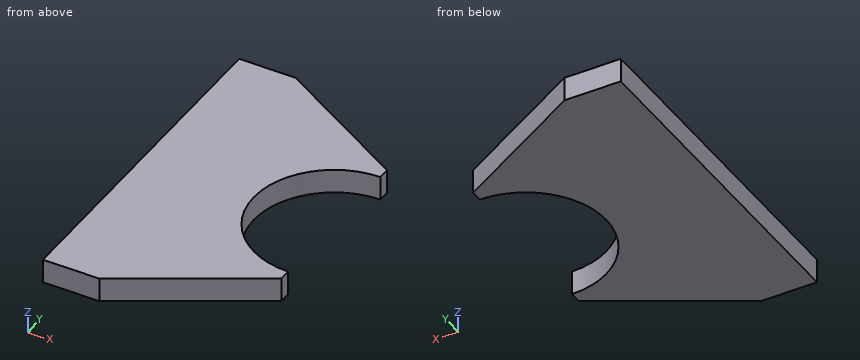
```python
from build123d import *

# Parameters (mm, degrees)
BOSS_EXTRUDE1_DEPTH = 3


with BuildPart() as part:
    # Sketch1 → Boss-Extrude1 (new, symmetric)
    with BuildSketch(Plane.XY):
        with BuildLine():
            Line((-48, -42.5), (-48, 42.5))
            Line((-48, 42.5), (-34, 42.5))
            Line((-34, 42.5), (0, 22.870090848))
            Line((0, 22.870090848), (0, 20))
            ThreePointArc((0, 20), (-20, 0), (0, -20))
            Line((0, -20), (0, -22.870090848))
            Line((0, -22.870090848), (-34, -42.5))
            Line((-34, -42.5), (-48, -42.5))
        make_face()
    extrude(amount=BOSS_EXTRUDE1_DEPTH, both=True)


solid = part.part
```
Geometry: final body of the model. Coordinates: model frame, mm. Coordinates: 2 decimals unless noted, no trailing zeros. Order: outer loops, then holes, each group sorted by start corner. A loop starts at its lowest first (then second) coordinate and runs counter-clockwise, first axis right, second up. Notation, with made-up numbers: (43.25, 12) -> (89.25, 12) arc R16 ccw to (89.25, 41) -> close; hole circle Ø2 at (4.5, -26). An arc over 180 degrees is marked (long way). Write item = value, one per line.
(1) Cut plane C-C on y = 0. Return loops of the section in (x, z), plus the area to 3 significant figures.
Solved:
outline = (-48, -3) -> (-20, -3) -> (-20, 3) -> (-48, 3) -> close
area = 168 mm²
(2) Cut plane B-B on x = -3.5. Return loops of the section in (y, z), plus the area to 3 significant figures.
Solved:
outline = (-24.89, -3) -> (-19.69, -3) -> (-19.69, 3) -> (-24.89, 3) -> close; (19.69, -3) -> (24.89, -3) -> (24.89, 3) -> (19.69, 3) -> close
area = 62.4 mm²
(3) Cut plane D-D on x = -29. Return loops of the section in (y, z), plus the area to 3 significant figures.
Solved:
outline = (-39.61, -3) -> (39.61, -3) -> (39.61, 3) -> (-39.61, 3) -> close
area = 475 mm²
(4) Cut plane A-A on z = -0.6. Return loops of the section in (x, y), plus the area to 3 significant figures.
Solved:
outline = (-48, -42.5) -> (-34, -42.5) -> (0, -22.87) -> (0, -20) arc R20 cw to (0, 20) -> (0, 22.87) -> (-34, 42.5) -> (-48, 42.5) -> close
area = 2,780 mm²
(5) Pin query (flat end, axial travel): pin 1 Ø2 at (y, z) = (29.5, -1) entering from +X; pin 2 Ø1 at (x, z) = (-30, -2) entering from +Y. Return the tip coordinate at first contact, or that it passes through.
Solved:
pin_1 = -9.75
pin_2 = 40.48
(6) Line query: line 1 (Y direction, x = -7, z = -0.75) (3 decimals); line 2 (Y direction, x = -9.5, z = -2.65); line 3 (X direction, y = 27.5, z = 0.3). Output: solid intervals per line, ascending.
Solved:
line_1 = -26.912 to -18.735, 18.735 to 26.912
line_2 = -28.35 to -17.6, 17.6 to 28.35
line_3 = -48 to -8.02
